The drawing under review shows one solid part. Ordinate dimensions are in mm from its lowest x, y, z. A direction names the side the tool comes from. Coordinates: 2 decimals unless noted, no trailing zeros. Order: outer loops, then holes, each group sorted by start corner. A loop starts at its lowest first (then second) coordinate and runs counter-clockwise, first axis right, second up. Notation, with made-up numbers: (2.5, 19.25) -> (54.5, 19.25) arc R18 ccw to (54.5, 40.25) -> close; hole circle Ø9 at (-38, -13.5). An arc over 180 degrees is marked (long way). Use one line per item in the form item = value.
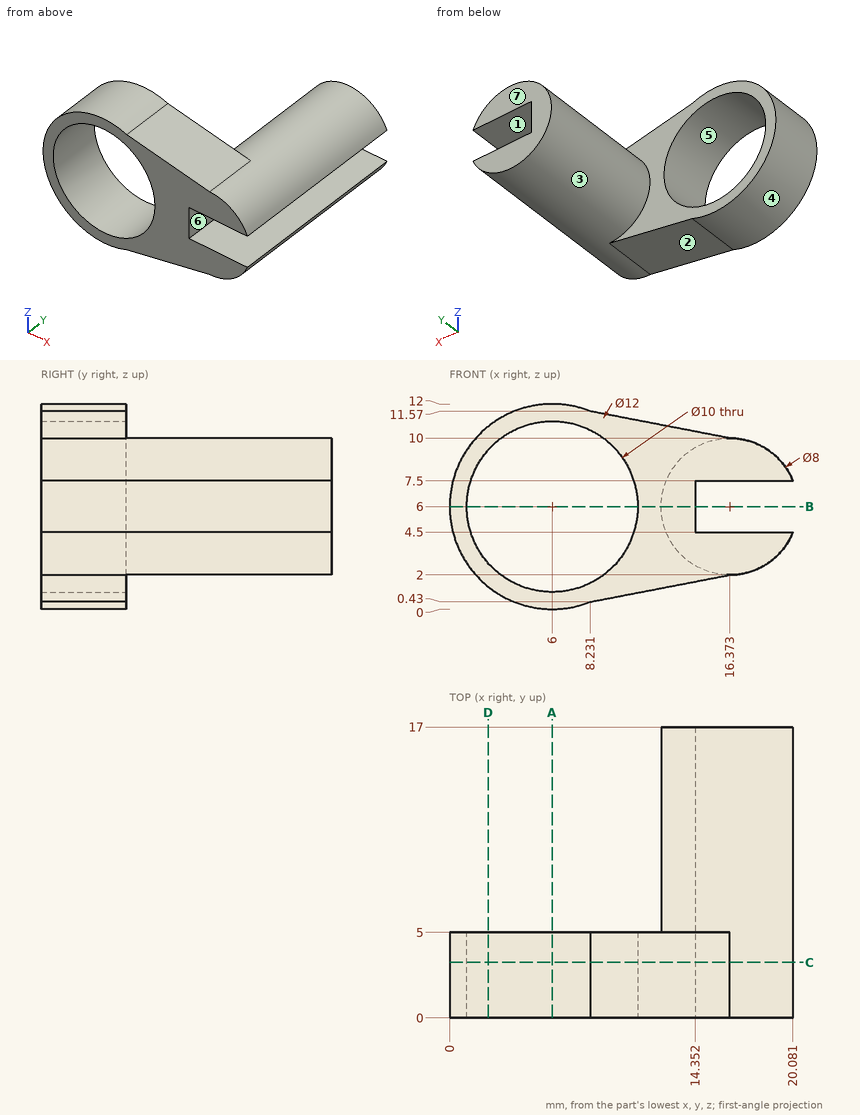
Item 1: Tool access review of the marked faces 1, 2 and 3: name each direction out of +Z, -Z, +X, -X, +Y, -Y from which nothing blocks a thin tool from reaching the whole face with its end or side.
Results found:
face_1 = +X, +Y, -Y
face_2 = -Z, +X, +Y, -Y
face_3 = +Y
Item 2: We need section B-B (z = 6). Write out the cut boundary in (x, y), plus the area to 3 significant figures.
Results found:
outline = (0, 0) -> (1, 0) -> (1, 5) -> (0, 5) -> close; (11, 0) -> (14.35, 0) -> (14.35, 17) -> (12.37, 17) -> (12.37, 5) -> (11, 5) -> close
area = 45.5 mm²
Item 3: We need section A-A (x = 6). Write out the cut boundary in (y, z).
Results found:
outline = (0, 0) -> (5, 0) -> (5, 1) -> (0, 1) -> close; (0, 11) -> (5, 11) -> (5, 12) -> (0, 12) -> close
Item 4: To check wall thickness, follow L1, parallel to Z at x = 6, y = 2.85; L2, parallel to Y at x = 1.25, z = 3.5; L3, parallel to X at y = 2, z = 8. State the ranges of each line that lie inside material, in increasing order. Write a range as from..to.
Results found:
L1 = 0..1, 11..12
L2 = 0..5
L3 = 0.34..1.42, 10.58..19.84
Item 5: We need section D-D (x = 2.25). Write out the cut boundary in (y, z).
Results found:
outline = (0, 1.32) -> (5, 1.32) -> (5, 2.69) -> (0, 2.69) -> close; (0, 9.31) -> (5, 9.31) -> (5, 10.68) -> (0, 10.68) -> close
Item 6: Clearance check with flat-ended pins moving along their axes: pin 1 (6 mm diameter, centred on x = 4.5, z = 3.5, fed in from +Y); pin 2 (6.5 mm diameter, centred on x = 18.5, y = 8.5, fed in from +Z); pin 3 (3 mm diameter, centred on x = 17.5, y = 11.5, fed in from -Z). State where each tip first meets the part, or that it passes through.
Results found:
pin_1 = 5
pin_2 = 10
pin_3 = 2
Item 7: Draft analysis for pull direction X (two halves, no side actions). For the marked faces 4, 5, 6 and 7, state which applies: released by +X, released by -X, zero draft, split by the parting line, or undercut.
Results found:
face_4 = split by the parting line
face_5 = undercut
face_6 = released by +X
face_7 = zero draft
Item 8: We need section C-C (y = 3.25). Write out the cut boundary in (x, z).
Results found:
outline = (8.23, 0.43) -> (16.37, 2) arc R4 ccw to (20.08, 4.5) -> (14.35, 4.5) -> (14.35, 7.5) -> (20.08, 7.5) arc R4 ccw to (16.37, 10) -> (8.23, 11.57) arc R6 ccw (long way) to start; hole circle Ø10 at (6, 6)
